Drawing for the job (mm, zero at the part's lowest x, y, z). A direction names the side the tool comes from. Coordinates: 2 decimals unless noted, no trailing zeros. Order: outer loops, then holes, each group sorted by start corner. A loop starts at its lowest first (then second) coordinate and runs counter-clockwise, first axis right, second up.
1) Mould opens along X. For the marked faces 1, 2, 3 and 4 say: +X half, -X half, draft (parallel to the pull), parting line (faces both ways), or undercut.
2) Tool access for the marked faces 5 and 6: list every direction of +Z, -Z, +X, -X, +Y, -Y with a clear straight run to the whole face (end or side of a thin tool).
3) Cut at C-C (y = 10.5). List the corners of the cut face in (x, z), and give its area (3 significant figures).
4) Wall check: L1, parallel to X at y = 7.25, z = 2.5; L2, parallel to Y at x = 6, z = 4.6; L3, parallel to Z at x = 21, y = 5.75. Give the ranges that are in metal, low to high.
5) Pin check, flat tips, straight feed: pin 1 Ø4 at (y, z) = (3.5, 15) entering from +X; pin 2 Ø3.5 at (x, y) = (33, 6.5) entering from +Z; pin 3 Ø2 at (y, z) = (5, 15.5) entering from -X. Stop position of each tip, or through.
6) Cut at A-A (x = 21). List the corners of the cut face in (y, z), and give its area (3 significant figures).
7) Cut at D-D (y = 5.25). List the corners of the cut face in (x, z), and give its area (3 significant figures).
8) Cut at B-B (z = 23). List the corners of the cut face in (x, y), and give its area (3 significant figures).
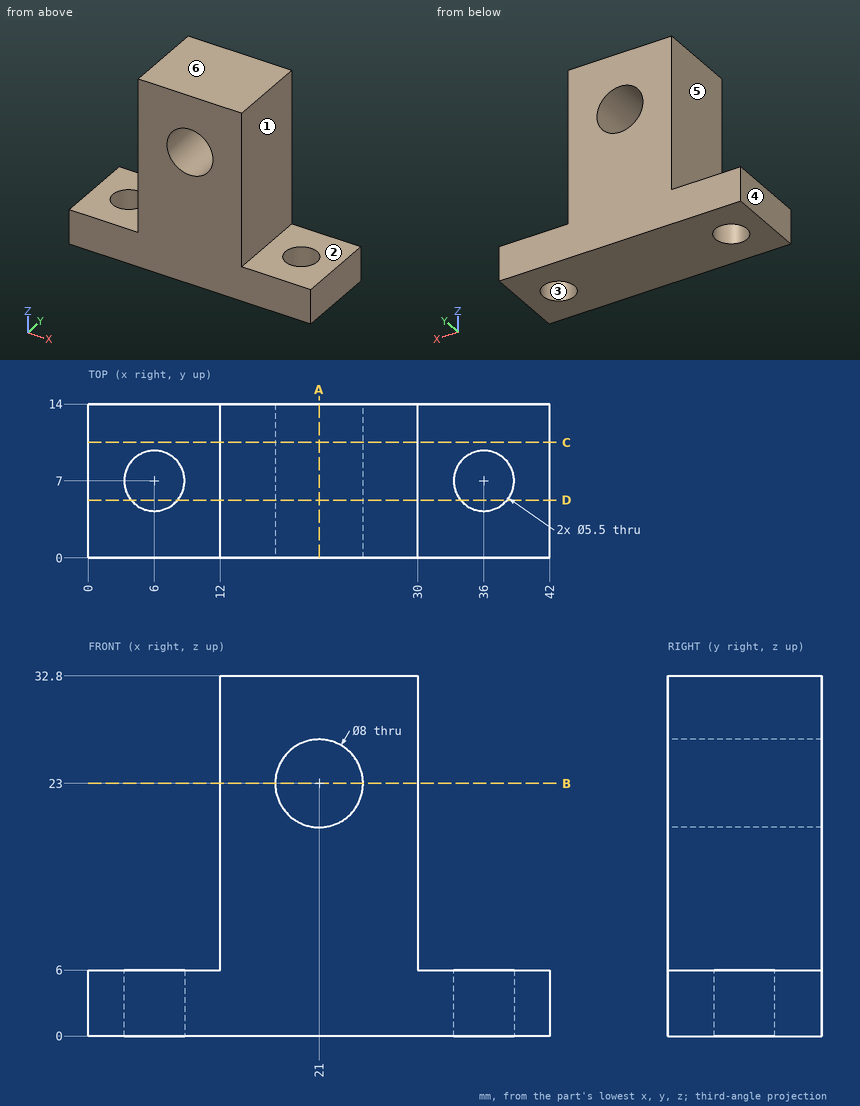
Geometry check:
1. face 1: +X half
1. face 2: draft
1. face 3: undercut
1. face 4: -X half
2. face 5: +Z, -X, +Y, -Y
2. face 6: +Z, +X, -X, +Y, -Y
3. outline: (0, 0) - (42, 0) - (42, 6) - (30, 6) - (30, 32.8) - (12, 32.8) - (12, 6) - (0, 6) - close; hole circle Ø8 at (21, 23)
3. area: 684 mm2
4. L1: x = 0 to 3.26, 8.74 to 33.26, 38.74 to 42
4. L2: y = 0 to 4.25, 9.75 to 14
4. L3: z = 0 to 19, 27 to 32.8
5. pin 1: stops at x = 30
5. pin 2: stops at z = 6
5. pin 3: stops at x = 12
6. outline: (0, 0) - (14, 0) - (14, 19) - (0, 19) - close; (0, 27) - (14, 27) - (14, 32.8) - (0, 32.8) - close
6. area: 347 mm2
7. outline: (0, 0) - (3.88, 0) - (3.88, 6) - (0, 6) - close; (8.12, 0) - (33.88, 0) - (33.88, 6) - (30, 6) - (30, 32.8) - (12, 32.8) - (12, 6) - (8.12, 6) - close; (38.12, 0) - (42, 0) - (42, 6) - (38.12, 6) - close; hole circle Ø8 at (21, 23)
7. area: 633 mm2
8. outline: (12, 0) - (17, 0) - (17, 14) - (12, 14) - close; (25, 0) - (30, 0) - (30, 14) - (25, 14) - close
8. area: 140 mm2
